from build123d import *

# Parameters (mm, degrees)
BOSS_EXTRUDE1_DEPTH = 21
FILLET1_R           = 1
CUT_EXTRUDE1_DEPTH  = 78.369244536


with BuildPart() as part:
    # Sketch1 → Boss-Extrude1 (new body)
    with BuildSketch(Plane(origin=(0, 0, 0), x_dir=(0, 0, -1), z_dir=(1, 0, 0))):
        Polygon((-34.5, 0), (-34.5, 28), (34.5, 28), (34.5, -28), (-34.5, -28), align=None)
    extrude(amount=BOSS_EXTRUDE1_DEPTH)

    # Fillet1
    fillet1_edges = [part.edges().sort_by_distance(p)[0] for p in [
        (21, 28, 0),
        (0, 28, 0),
    ]]
    fillet(fillet1_edges, radius=FILLET1_R)

    # Sketch2 → Cut-Extrude1 (cut, through all)
    with BuildSketch(Plane(origin=(0, 0, -34.5), x_dir=(-1, 0, 0), z_dir=(0, 0, -1))):
        with BuildLine():
            Line((-21, -4.5), (-19, -4.5))
            ThreePointArc((-19, -4.5), (-16.5, -7), (-14, -4.5))
            Line((-14, -4.5), (-14, 4.5))
            ThreePointArc((-14, 4.5), (-16.5, 7), (-19, 4.5))
            Line((-19, 4.5), (-21, 4.5))
            Line((-21, 4.5), (-21, -4.5))
        make_face()
    extrude(amount=-CUT_EXTRUDE1_DEPTH, mode=Mode.SUBTRACT)


solid = part.part
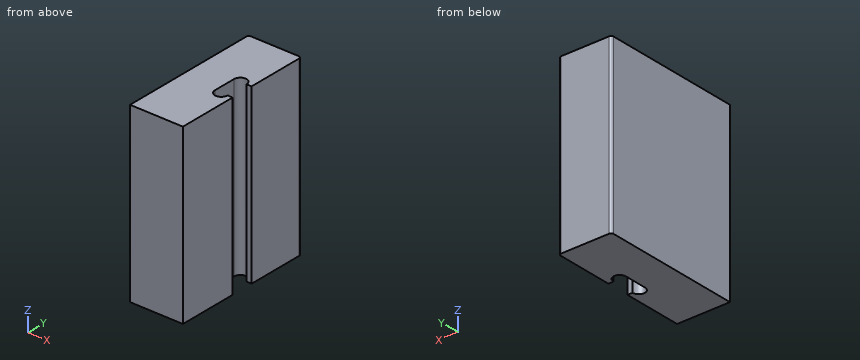
Can you work these out from the model? Positions are in its coordinate system, mm. Round coordinates to 2 decimals unless told otherwise and drop trailing zeros. Write each loop counter-clockwise with the first axis right and the second up, starting at its lowest first coordinate (ties: lowest second). Pieces come first, ordered by that corner, then holes. Notation, with made-up numbers: M -13.5,-34 L -3.5,-34 A29 cw -3.5,2 Z; hole C 29.25,-5.75 d4. An arc over 180 degrees is marked long. Use a Markdown table: item, result.
Item 1: I want a section at A-A (z = -11.5). List the corners of the cut face in (x, y) for me, and give its area (3 significant figures).
Found:
| item | result |
|---|---|
| outline | M 0,-28 L 21,-28 L 21,-4.5 L 19,-4.5 A2.5 cw 14,-4.5 L 14,4.5 A2.5 cw 19,4.5 L 21,4.5 L 21,27 A1 ccw 20,28 L 1,28 A1 ccw 0,27 Z |
| area | 1,090 mm2 |
Item 2: If I drill on line 1 along Y through (x, z) = (20, -30); line 2 along X through (y, z) = (-3.5, 14.5); line 3 along X through (y, z) = (-5.5, 13), over which ranges is the centre line in solid material (lowest first)? Write a range as [from, to].
Found:
| item | result |
|---|---|
| line 1 | y = [-28, -4.5], [4.5, 28] |
| line 2 | x = [0, 14] |
| line 3 | x = [0, 14.21], [18.79, 21] |
Item 3: I want a section at B-B (x = 16.5). List the corners of the cut face in (y, z) for me, and give its area (3 significant figures).
Found:
| item | result |
|---|---|
| outline | M -28,-34.5 L -7,-34.5 L -7,34.5 L -28,34.5 Z; M 7,-34.5 L 28,-34.5 L 28,34.5 L 7,34.5 Z |
| area | 2,900 mm2 |
